Autodesk Fusion 360 part; units mm, degrees
sketch "Sketch4" plane through (0, 0, 0) normal (0, 1, 0) x (1, 0, 0)
  circle A0 centre (0, 0) radius 2.625
  circle A1 centre (0, 0) radius 5.625
  line L0 (-5.625, 0) -> (-5.625, -32)
  line L1 (-5.625, -32) -> (-0.875, -32)
  line L2 (1.375, -28.5) -> (1.375, -5.4544)
  line L3 (5.1055, 2.361) -> (1.6179, 13.0978)
  line L4 (-0.9022, 14.3821) -> (0.2867, 14.7683)
  line L5 (-0.9976, 12.2483) -> (0.7348, 6.9151)
  line L6 (1.375, -28.5) -> (2.3896, -28.4915)
  line L7 (2.3896, -28.4915) -> (3.875, -8.23)
  line L8 (3.875, -8.23) -> (5.975, -8.23)
  line L9 (5.975, -8.23) -> (5.975, -10.03)
  line L10 (5.975, -10.03) -> (5.0465, -10.03)
  line L11 (5.0465, -10.03) -> (3.6939, -28.4805)
  line L12 (3.6939, -28.4805) -> (2.3896, -28.4915)
  line L13 (1.375, -28.5) -> (1.3456, -25.0001)
  line L14 (1.3456, -25.0001) -> (2.6456, -25.0001)
  arc A2 (0.2867, 14.7683) -> (-0.9976, 12.2483) centre (0.9046, 12.8661) ccw
  arc A3 (1.6179, 13.0978) -> (-0.9022, 14.3821) centre (-0.2843, 12.48) ccw
  line L15 (0, 5.625) -> (0.0926, 5.6551)
  arc A4 (0.0926, 5.6551) -> (0.7348, 6.9151) centre (-0.2163, 6.6062) ccw
  line L16 (-5.625, -32) -> (-0.875, -32)
  line L17 (-0.875, -32) -> (-0.875, -28.5)
  line L18 (-0.875, -28.5) -> (1.375, -28.5)
  dimension "d17" = 5.25
  dimension "d18" = 11.25
  dimension "d19" = 32
  dimension "d23" = 3.5
  dimension "d24" = 18.5
  dimension "d25" = 1.8
  dimension "d26" = 2.1
  dimension "d28" = 1.3
  dimension "d29" = 1.3
  dimension "d30" = 2.5
  dimension "d31" = 2
  dimension "d32" = 2.75
  dimension "d33" = 1
  dimension "d34" = 4.75
  dimension "d35" = 3.5
  dimension "d39" = 7
extrude "Extrude1" add sketch "Sketch4" along normal blind 4.6 contours A1 | A1 L3 L5 A2 A3 L15 A4 | A1 L0 L1 L2 L13 L14 L16 L17 L18 | L2 L6 L7 L14 | L2 L13 L14 | L7 L8 L9 L10 L11 L12
sketch "Sketch5" plane through (0, 0, 0) normal (0, -1, 0) x (1, 0, 0)
  circle A0 centre (0, 0) radius 2.625
  arc A1 (-5.625, 0) -> (0, -5.625) centre (0, 0) ccw
  line L0 (0, -5.625) -> (0.0926, -5.6551)
  arc A2 (0.7348, -6.9151) -> (0.0926, -5.6551) centre (-0.2163, -6.6062) ccw
  line L1 (0.7348, -6.9151) -> (-0.9976, -12.2483)
  arc A3 (-0.9976, -12.2483) -> (-0.2768, -14.4799) centre (0.9046, -12.8661) ccw
  arc A4 (-0.2768, -14.4799) -> (1.6179, -13.0978) centre (-0.2843, -12.48) ccw
  line L2 (1.6179, -13.0978) -> (5.1055, -2.361)
  arc A5 (5.1055, -2.361) -> (1.375, 5.4544) centre (0, 0) ccw
  line L3 (1.375, 5.4544) -> (1.375, 25.0001)
  line L4 (1.375, 25.0001) -> (2.6456, 25.0001)
  line L5 (2.6456, 25.0001) -> (3.875, 8.23)
  line L6 (3.875, 8.23) -> (5.975, 8.23)
  line L7 (5.975, 8.23) -> (5.975, 10.03)
  line L8 (5.975, 10.03) -> (5.0465, 10.03)
  line L9 (5.0465, 10.03) -> (3.6939, 28.4805)
  line L10 (-0.875, 28.5) -> (-0.875, 32)
  line L11 (-0.875, 32) -> (-5.625, 32)
  line L12 (-5.625, 32) -> (-5.625, 0)
  line L13 (-5.625, 26.6) -> (-5.625, 32)
  line L14 (-5.625, 32) -> (4.875, 32)
  line L15 (4.875, 32) -> (4.875, 26)
  line L16 (-5.625, 26.6) -> (4.875, 26.6)
  line L17 (4.875, 26.6) -> (4.875, 26)
  line L18 (3.6939, 28.4805) -> (1.375, 28.5)
  line L19 (1.375, 28.5) -> (-0.875, 28.5)
  dimension "d42" = 10.5
  dimension "d59" = 5.4
extrude "Extrude2" add sketch "Sketch5" along normal blind 9.25 contours L9 L10 L11 L12 L13 L14 L16 L18 L19 | L9 L10 L14 L15 L16 L18 L19
sketch "Sketch7" plane through (0, -9.25, 0) normal (0, -1, 0) x (1, 0, 0)
  line L0 (-5.625, 26.6) -> (4.875, 26.6)
  line L1 (4.875, 26.6) -> (4.875, 32)
  line L2 (4.875, 32) -> (-5.625, 32)
  line L3 (-5.625, 32) -> (-5.625, 26.6)
  line L4 (-5.625, 32) -> (3.625, 32)
  line L5 (3.625, 32) -> (3.625, 26.6)
  line L6 (3.625, 26.6) -> (-5.625, 26.6)
  line L7 (-5.625, 26.6) -> (-5.625, 32)
  dimension "d43" = 9.25
  dimension "d58" = 5.4
extrude "Extrude3" add sketch "Sketch7" along normal blind 29 contours L0 L2 L3 L4 L5 L6 L7
sketch "Sketch8" plane through (0, -38.25, 0) normal (0, -1, 0) x (1, 0, 0)
  line L0 (-5.625, 26.6) -> (3.625, 26.6)
  line L1 (3.625, 26.6) -> (3.625, 32)
  line L2 (3.625, 32) -> (-5.625, 32)
  line L3 (-5.625, 32) -> (-5.625, 26.6)
  line L4 (3.625, 32) -> (-2.675, 32)
  line L5 (-2.675, 32) -> (-2.675, 25.81)
  line L6 (-2.675, 25.81) -> (3.625, 25.81)
  line L7 (3.625, 25.81) -> (3.625, 32)
  dimension "d46" = 6.3
extrude "Extrude4" add sketch "Sketch8" along normal blind 15.75 contours L0 L1 L2 L4 L5 L7
mirror "Mirror1" about plane through (0, -54, 0) normal (0, -1, 0) of bodies 1 merged
chamfer "Chamfer1" distance 2.95 angle 45 2 edges at (-2.675, -69.75, 29.3) (-2.675, -38.25, 29.3)
fillet "Fillet1" radius 1 4 edges at (-0.875, 0, 30.25) (0.25, 0, 28.5) (2.5345, 0, 28.4903) (-0.875, 2.3, 28.5)
fillet "Fillet2" radius 1 4 edges at (-0.875, -110.3, 28.5) (2.5345, -108, 28.4903) (0.25, -108, 28.5) (-0.875, -108, 30.25)
fillet "Fillet3" radius 1 2 edges at (3.625, -98.75, 29.3) (3.625, -9.25, 29.3)
fillet "Fillet4" radius 0.5 2 edges at (-0.8966, 0, 26.6) (-0.8966, -108, 26.6)
equation "d47 = 27 mm - 11.25 mm"
Input: part model. Units: mm. Frame: model coordinates. A direction names the side the tool comes from. Give positions to 0.01 mm unless a question says otherwise; leave off trailing zeros. Loops run counter-clockwise (first coordinate to the right, second up) from the corner with the lowest first, then second, coordinate; pieces in that order, holes last. Notation, with made-up numbers: (-29.75, 18.5) - (19.25, 18.5) arc R18 cw to (19.25, 50.5) - close; hole circle Ø9 at (40, 67). An arc over 180 degrees is marked (long way). Use CSV: the item, a comma, the result in double quotes. Start each with the question number.
Item 1: Section B-B on z = 18.5. Return loops of the section in (x, y) (3 decimals), then the cut area to 3 significant figures.
Item 2: Contact query for flat-ended pins moving along their axis: P1, Ø3, axis at y = -111.5, z = 30.5, coming from the +X side; P2, Ø6, axis at y = -54, z = 29, coming from the -X side (3 decimals); P3, Ø1, axis at x = 2, y = -111, coming from the -Z side. Output: stop coordinate, or through.
Item 3: Section D-D on y = -101. Return loops of the section in (x, z) (3 decimals).
Item 4: Line query: line 1 (Y direction, x = 0.75, z = 21.5); line 2 (X direction, y = -109, z = 0) (3 decimals); line 3 (Z direction, x = 0, y = -64). Output: solid intervals per line, ascending.
Item 5: Section A-A on z = -11. Return loops of the section in (x, y).
Item 6: Section C-C on y = -64.5. Return loops of the section in (x, z) (3 decimals), then the cut area to 3 significant figures.
Item 7: Mould query, pull axis Y, two halves, no side actions, for faces 1 (the flat face through (-1, 4.6, 8)), 2 (the flat face through (-2.675, -54, 29)), 3 (the flat face through (4.324, -110.014, 19.892)). Classes: pulls with the +Y half, pulls with the -Y half, needs draft (parallel to the pull), parting line crosses it, or undercut.
Item 8: Reachability of faces 4 (the flat face through (1.375, -110, 15)), 5 (the flat face through (5, -110, 8.23)), 6 (the flat face through (-0.119, -110.268, -9.544)) from +Z, -Z, +X, -X, +Y, -Y: full face, straight path, thin tool, end or side. Return the list, or none.
Ans:
1,outline,"(-5.625, -112.6) - (1.375, -112.6) - (1.375, -108) - (-5.625, -108) - close; (-5.625, 0) - (1.375, 0) - (1.375, 4.6) - (-5.625, 4.6) - close; (3.122, -112.6) - (4.426, -112.6) - (4.426, -108) - (3.122, -108) - close; (3.122, 0) - (4.426, 0) - (4.426, 4.6) - (3.122, 4.6) - close"
1,area,"76.4 mm2"
2,P1,"stops at x = -0.74"
2,P2,"stops at x = -2.675"
2,P3,"stops at z = -13.38"
3,outline,"(-5.625, 26.6) - (4.875, 26.6) - (4.875, 32) - (-5.625, 32) - close"
4,line 1,"y = -112.6 to -108, 0 to 4.6"
4,line 2,"x = -5.625 to -2.625, 2.625 to 5.625"
4,line 3,"z = 26.6 to 32"
5,outline,"(-0.59, -112.6) - (2.3, -112.6) - (2.3, -108) - (-0.59, -108) - close; (-0.59, 0) - (2.3, 0) - (2.3, 4.6) - (-0.59, 4.6) - close"
6,outline,"(-2.675, 26.6) - (3.625, 26.6) - (3.625, 32) - (-2.675, 32) - close"
6,area,"34.0 mm2"
7,face 1,"pulls with the +Y half"
7,face 2,"undercut"
7,face 3,"needs draft"
8,face 4,"+Y, -Y"
8,face 5,"+X, +Y, -Y"
8,face 6,"-X, +Y, -Y"
